```python
from build123d import *

# Parameters (mm, degrees)
BOSS_EXTRUDE1_DEPTH = 2
SKETCH3_W           = 1.47
SKETCH3_H           = 33
BOSS_EXTRUDE3_DEPTH = 0.1
SKETCH4_W           = 11.437084048
SKETCH4_H           = 43
BOSS_EXTRUDE4_DEPTH = 0.5
SKETCH5_R           = 3.25
BOSS_EXTRUDE5_DEPTH = 1
BOSS_EXTRUDE6_DEPTH = 0.7
CUT_EXTRUDE2_DEPTH  = 10
FILLET4_R           = 1
SKETCH7_R           = 1.432474787
BOSS_EXTRUDE7_DEPTH = 0.7


with BuildPart() as part:
    # Sketch1 → Boss-Extrude1 (new body)
    with BuildSketch(Plane(origin=(0, 0, 0), x_dir=(1, 0, 0), z_dir=(0, 1, 0))):
        with BuildLine():
            Line((-26.5, 21.5), (-31.5, 21.5))
            Line((-31.5, 21.5), (-31.5, 16.5))
            Line((-31.5, 16.5), (-31.5, -16.5))
            Line((-31.5, -16.5), (-31.5, -21.5))
            Line((-31.5, -21.5), (-26.5, -21.5))
            Line((-26.5, -21.5), (26.5, -21.5))
            ThreePointArc((26.5, -21.5), (30.035533906, -20.035533906), (31.5, -16.5))
            Line((31.5, -16.5), (31.5, 16.5))
            ThreePointArc((31.5, 16.5), (30.035533906, 20.035533906), (26.5, 21.5))
            Line((26.5, 21.5), (-26.5, 21.5))
        make_face()
    extrude(amount=BOSS_EXTRUDE1_DEPTH)

    # Sketch3 → Boss-Extrude3 (add)
    with BuildSketch(Plane(origin=(0, 0, 0), x_dir=(1, 0, 0), z_dir=(0, 1, 0))):
        with Locations((32.235, 0)):
            Rectangle(SKETCH3_W, SKETCH3_H)
    extrude(amount=BOSS_EXTRUDE3_DEPTH)

    # Sketch4 → Boss-Extrude4 (add)
    with BuildSketch(Plane.XZ):
        with Locations((20.781457976, 0)):
            Rectangle(SKETCH4_W, SKETCH4_H)
    extrude(amount=BOSS_EXTRUDE4_DEPTH)

    # Sketch5 → Boss-Extrude5 (add)
    with BuildSketch(Plane.XZ.offset(0.5)):
        with Locations((20.781457976, -10.75)):
            Circle(SKETCH5_R)
        with Locations((20.781457976, 0)):
            Circle(SKETCH5_R)
        with Locations((20.781457976, 10.75)):
            Circle(SKETCH5_R)
    extrude(amount=BOSS_EXTRUDE5_DEPTH)

    # Sketch6 → Boss-Extrude6 (add)
    with BuildSketch(Plane.XZ.offset(1.5)):
        Polygon((22.728056174, 9.551943968), (20.845705836, 13.034831506), (18.770611919, 9.663224526), align=None)
        Polygon((20.781457976, -2.122654215), (22.61973045, 1.061327108), (18.943185502, 1.061327108), align=None)
    extrude(amount=BOSS_EXTRUDE6_DEPTH)

    # Sketch9 → Cut-Extrude2 (cut)
    with BuildSketch(Plane(origin=(0, 0, 0), x_dir=(-1, 0, 0), z_dir=(0, -1, 0))):
        with BuildLine():
            Line((-5.062915952, 16.5), (21.5, 16.5))
            ThreePointArc((21.5, 16.5), (25.035533906, 15.035533906), (26.5, 11.5))
            Line((26.5, 11.5), (26.5, -11.5))
            ThreePointArc((26.5, -11.5), (25.035533906, -15.035533906), (21.5, -16.5))
            Line((21.5, -16.5), (-5.062915952, -16.5))
            ThreePointArc((-5.062915952, -16.5), (-8.598449858, -15.035533906), (-10.062915952, -11.5))
            Line((-10.062915952, -11.5), (-10.062915952, 11.5))
            ThreePointArc((-10.062915952, 11.5), (-8.598449858, 15.035533906), (-5.062915952, 16.5))
        make_face()
    extrude(amount=-CUT_EXTRUDE2_DEPTH, mode=Mode.SUBTRACT)

    # Fillet4
    fillet4_edges = [part.edges().sort_by_distance(p)[0] for p in [
        (8.598449858, 0, 15.035533906),
        (-8.218542024, 0, 16.5),
        (-25.035533906, 0, 15.035533906),
        (-26.5, 0, 0),
        (-25.035533906, 0, -15.035533906),
        (-8.218542024, 0, -16.5),
        (8.598449858, 0, -15.035533906),
        (10.062915952, 0, 0),
    ]]
    fillet(fillet4_edges, radius=FILLET4_R)

    # Sketch7 → Boss-Extrude7 (add)
    with BuildSketch(Plane(origin=(0, -1.5, 0), x_dir=(-1, 0, 0), z_dir=(0, -1, 0))):
        with Locations((-20.781457976, 10.75)):
            Circle(SKETCH7_R)
    extrude(amount=BOSS_EXTRUDE7_DEPTH)


solid = part.part
```
The model under review builds one solid part; all positions refer to its coordinate system, in mm. A direction names the side the tool comes from. Round coordinates to 2 decimals unless told otherwise and drop trailing zeros. Loops run counter-clockwise (first coordinate to the right, second up) from the corner with the lowest first, then second, coordinate; pieces in that order, holes last.
1) Tool access review of faces 4 (the face through (31.5, 1, 0)), 5 (the face through (21.8, -1.85, 11.27)), 6 (the face through (17.535, -0.993, 10.893)): name each direction out of +Z, -Z, +X, -X, +Y, -Y from which nothing blocks a thin tool from reaching the whole face with its end or side.
Values follow:
face 4: +Z, -Z, +X, +Y
face 5: +Z, +X, -Y
face 6: -Y
2) The part is to be moulded in two halves that separate along Z. For faces 1 (the face through (30, 0.99, 20.07)), 2 (the face through (-9, 0, 19)), 3 (the face through (8.637, 1.493, -14.996)), say which applies: pulls with the +Z half, pulls with the -Z half, needs draft (parallel to the pull), parting line crosses it, or undercut.
Values follow:
face 1: pulls with the +Z half
face 2: needs draft
face 3: undercut
3) Wall thickness on line 1 along X through (y, z) = (1.15, 1); line 2 along Z through (x, y) = (20, -1.95); line 3 along Y through (x, z) = (30, -14): over which ranges is each line inside the solid? List them lowest first.
Values follow:
line 1: x = -31.5 to -26.5, 10.06 to 31.5
line 2: z = -11.95 to -9.55, -0.77 to 1.06, 9.63 to 11.66
line 3: y = 0 to 2
4) Consider section C-C on z = 10.75. State the section outline as (x, y) points, then the cut area to 3 significant figures.
Values follow:
outline: (-31.5, 0) - (-27.5, 0) arc R1 ccw to (-26.5, 1) - (-26.5, 2) - (-31.5, 2) - close; (10.06, 1) arc R1 ccw to (11.06, 0) - (15.06, 0) - (15.06, -0.5) - (17.53, -0.5) - (17.53, -1.5) - (19.44, -1.5) - (19.44, -2.2) - (22.08, -2.2) - (22.08, -1.5) - (24.03, -1.5) - (24.03, -0.5) - (26.5, -0.5) - (26.5, 0) - (32.97, 0) - (32.97, 0.1) - (31.5, 0.1) - (31.5, 2) - (10.06, 2) - close
area: 66.7 mm2
5) Consider section A-A on z = -10.75. State the section outline as (x, y) points.
Values follow:
outline: (-31.5, 0) - (-27.5, 0) arc R1 ccw to (-26.5, 1) - (-26.5, 2) - (-31.5, 2) - close; (10.06, 1) arc R1 ccw to (11.06, 0) - (15.06, 0) - (15.06, -0.5) - (17.53, -0.5) - (17.53, -1.5) - (19.35, -1.5) - (19.35, -2.2) - (22.21, -2.2) - (22.21, -1.5) - (24.03, -1.5) - (24.03, -0.5) - (26.5, -0.5) - (26.5, 0) - (32.97, 0) - (32.97, 0.1) - (31.5, 0.1) - (31.5, 2) - (10.06, 2) - close
6) Clearance check with flat-ended pins moving along their axes: P1, Ø7, axis at x = 29, z = 8.5, coming from the -Y side; P2, Ø0.5, axis at y = 1.5, z = 3.5, coming from the +X side; P3, Ø3.5, axis at x = 22.5, z = 6.5, coming from the -Y side. State where each tip first meets the part, or that it passes through.
Values follow:
P1: stops at y = -0.5
P2: stops at x = 31.5
P3: stops at y = -1.5
7) Consider section B-B on x = -16.5. State the section outline as (y, z) points, then the cut area to 3 significant figures.
Values follow:
outline: (0, -21.5) - (2, -21.5) - (2, -16.5) - (1, -16.5) arc R1 ccw to (0, -17.5) - close; (0, 17.5) arc R1 ccw to (1, 16.5) - (2, 16.5) - (2, 21.5) - (0, 21.5) - close
area: 19.6 mm2
